Check sheet for the modelled part. Datum: model origin and axes. Units: mm. Face numbers are marked on the shaded views. A direction names the side the tool comes from. Round coordinates to 2 decimals unless told otherwise and drop trailing zeros. Write each loop counter-clockwise with the first axis right and the second up, starting at its lowest first coordinate (ties: lowest second). Pieces come first, ordered by that corner, then holes. Notation, with made-up numbers: (52.5, 26) - (58.5, 26) arc R18 ccw to (58.5, 32) - close; hole circle Ø5 at (-23.75, 89). An arc over 180 degrees is marked (long way). Answer as a JSON object with one key per item and string values. Group by question number.
Item 1: Thickness scan on line 1 (X direction, y = 1.3, z = 0); line 2 (Y direction, x = 9, z = -13.5); line 3 (Z direction, x = -16.5, y = 1.25). Record the ranges inside material, lowest first.
Item 2: Sectioned sample at B-B on z = -4. Record the boundary of the cut face in (x, y).
Item 3: Sectioned sample at D-D on y = 7. Record the boundary of the cut face in (x, z), plus the area to 3 significant figures.
Item 4: Sectioned sample at C-C on x = 15.5. Record the boundary of the cut face in (y, z).
Item 5: Set-up check for the marked faces 1 and 2: record each of +Z, -Z, +X, -X, +Y, -Y from which the full face is reachable in a straight line by a thin tool's end or side.
Item 6: Sectioned sample at A-A on x = 0. Record the boundary of the cut face in (y, z).
Item 7: Gauge pin test, flat ends, axial feed: P1, Ø5, axis at x = 7.5, y = 14, coming from the -Z side; P2, Ø1, axis at x = 4.5, z = -10.5, coming from the +Y side. Record the tip position at first contact, or that the pin passes through.
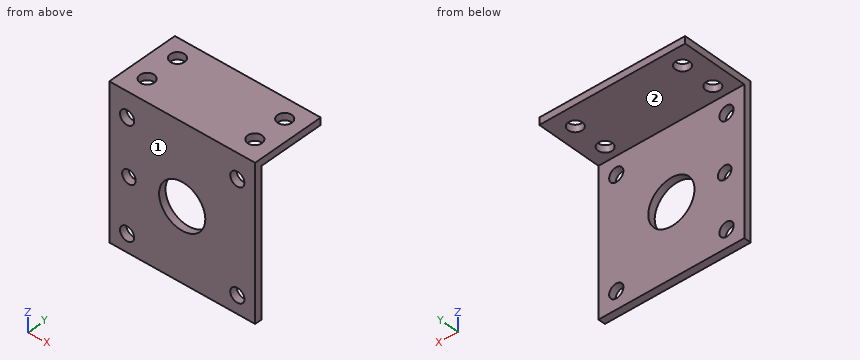
```python
from build123d import *

# Parameters (mm, degrees)
SKETCH1_W           = 41
SKETCH1_H           = 41
SKETCH1_R           = 2
SKETCH1_R_2         = 6.5
BOSS_EXTRUDE1_DEPTH = 2
SKETCH2_W           = 41
SKETCH2_H           = 20.5
BOSS_EXTRUDE2_DEPTH = 2
SKETCH3_R           = 2
CUT_EXTRUDE1_DEPTH  = 10
SKETCH6_R           = 1.911397566
CUT_EXTRUDE4_DEPTH  = 10


with BuildPart() as part:
    # Sketch1 → Boss-Extrude1 (new body)
    with BuildSketch(Plane(origin=(0, 0, 0), x_dir=(1, 0, 0), z_dir=(0, 1, 0))):
        Rectangle(SKETCH1_W, SKETCH1_H)
        with Locations(Location((-15.5, -15.5, 0), (0, 0, 270))):
            Circle(SKETCH1_R, mode=Mode.SUBTRACT)
        with Locations(Location((-15.5, 15.5, 0), (0, 0, 270))):
            Circle(SKETCH1_R, mode=Mode.SUBTRACT)
        with Locations(Location((15.5, 15.5, 0), (0, 0, 270))):
            Circle(SKETCH1_R, mode=Mode.SUBTRACT)
        with Locations(Location((0, 0, 0), (0, 0, 270))):
            Circle(SKETCH1_R_2, mode=Mode.SUBTRACT)
        with Locations(Location((15.5, -15.5, 0), (0, 0, 270))):
            Circle(SKETCH1_R, mode=Mode.SUBTRACT)
    extrude(amount=BOSS_EXTRUDE1_DEPTH)

    # Sketch2 → Boss-Extrude2 (add)
    with BuildSketch(Plane.XY.offset(20.5)):
        with Locations((0, 10.25)):
            Rectangle(SKETCH2_W, SKETCH2_H)
    extrude(amount=BOSS_EXTRUDE2_DEPTH)

    # Sketch3 → Cut-Extrude1 (cut)
    with BuildSketch(Plane(origin=(0, 0, 20.5), x_dir=(-1, 0, 0), z_dir=(0, 0, -1))):
        with Locations((-15.161511711, 5.844100373)):
            Circle(SKETCH3_R)
        with Locations((15.146476182, 15.353198296)):
            Circle(SKETCH3_R)
        with Locations(Location((-15.210908875, 15.130767232, 0), (0, 0, 180))):
            Circle(SKETCH3_R)
        with Locations(Location((15.196521792, 5.944623662, 0), (0, 0, 180))):
            Circle(SKETCH3_R)
    extrude(amount=-CUT_EXTRUDE1_DEPTH, mode=Mode.SUBTRACT)

    # Sketch6 → Cut-Extrude4 (cut)
    with BuildSketch(Plane(origin=(0, 0, 0), x_dir=(-1, 0, 0), z_dir=(0, -1, 0))):
        with Locations(Location((14.973447389, 0.105568023, 0), (0, 0, 90))):
            Circle(SKETCH6_R)
    extrude(amount=-CUT_EXTRUDE4_DEPTH, mode=Mode.SUBTRACT)


solid = part.part
```
Completed:
{
 "1": {"line 1": "-20.5 to -16.88, -13.06 to -6.5, 6.5 to 20.5", "line 2": "0 to 2", "line 3": "-20.5 to -17.23, -13.77 to -1.26, 1.04 to 13.77, 17.23 to 22.5"},
 "2": {"outline": "(-20.5, 0) - (-5.12, 0) - (-5.12, 2) - (-20.5, 2) - close; (5.12, 0) - (20.5, 0) - (20.5, 2) - (5.12, 2) - close"},
 "3": {"outline": "(-20.5, 20.5) - (-16.9, 20.5) - (-16.9, 22.5) - (-20.5, 22.5) - close; (-13.5, 20.5) - (13.53, 20.5) - (13.53, 22.5) - (-13.5, 22.5) - close; (16.79, 20.5) - (20.5, 20.5) - (20.5, 22.5) - (16.79, 22.5) - close", "area": "68.7 mm²"},
 "4": {"outline": "(0, -20.5) - (2, -20.5) - (2, -17.5) - (0, -17.5) - close; (0, -13.5) - (2, -13.5) - (2, 13.5) - (0, 13.5) - close; (0, 17.5) - (2, 17.5) - (2, 20.5) - (3.87, 20.5) - (3.87, 22.5) - (0, 22.5) - close; (7.82, 20.5) - (13.15, 20.5) - (13.15, 22.5) - (7.82, 22.5) - close; (17.11, 20.5) - (20.5, 20.5) - (20.5, 22.5) - (17.11, 22.5) - close"},
 "5": {"face 1": "+Z, -Z, +X, -X, -Y", "face 2": "-Z, +X, -X, +Y"},
 "6": {"outline": "(0, -20.5) - (2, -20.5) - (2, -6.5) - (0, -6.5) - close; (0, 6.5) - (2, 6.5) - (2, 20.5) - (20.5, 20.5) - (20.5, 22.5) - (0, 22.5) - close"},
 "7": {"P1": "z = 20.5", "P2": "y = 2"}
}
